The model under review builds one solid part; all positions refer to its coordinate system, in mm. Round coordinates to 2 decimals unless told otherwise and drop trailing zeros. Write each loop counter-clockwise with the first axis right and the second up, starting at its lowest first coordinate (ties: lowest second). Pieces come first, ordered by that corner, then holes. Notation, with made-up numbers: (40, 24) -> (98, 24) arc R14 ccw to (98, 41) -> close; hole circle Ø11 at (35, 86.25). An arc over 180 degrees is marked (long way). Answer as a JSON object with one key per item and string values. Group by question number.
1) We need section A-A, the plane x = -25.75. Write out the cut boundary in (y, z).
2) Mouldability with a two-part tool opening along X and no side actions: class faces 1 (the flat face through (30, 0, 1)), 2 (the flat face through (-14, 14, 2)), 3 (the cylindrical face through (-2.343, -17.847, 0.986)) as pulls with the +X half, pulls with the -X half, needs draft (parallel to the pull), parting line crosses it, or undercut.
3) To check wall thickness, follow probe 1 along Y at (x, z) = (-25.75, 0.5); probe 2 along X at (y, z) = (-26.5, 0.6); probe 3 along Y at (x, z) = (0, 1.4). State the ranges of each line that lie inside material, in increasing order. Write a range as [from, to].
4) We need section B-B, the plane z = 1.25. Write out the cut boundary in (x, y).
5) We need section D-D, the plane x = 0. Write out the cut boundary in (y, z).
Autodesk Fusion 360 part; units mm, degrees
sketch "Sketch1" plane through (0, 0, 0) normal (0, 0, 1) x (1, 0, 0)
  line L0 (-30, 30) -> (30, 30)
  line L1 (30, 30) -> (30, -30)
  line L2 (30, -30) -> (-30, -30)
  line L3 (-30, -30) -> (-30, 30)
  line L4 (-30, 30) -> (30, -30) construction
  line L5 (30, 30) -> (-30, -30) construction
  circle A0 centre (-25.75, 25.75) radius 1.55
  circle A1 centre (25.75, 25.75) radius 1.55
  circle A2 centre (25.76, -25.76) radius 1.55
  circle A3 centre (-25.75, -25.75) radius 1.55
  circle A4 centre (0, 0) radius 18
  dimension "d1" = 60
  dimension "d2" = 60
  dimension "d3" = 3.1
  dimension "d4" = 3.1
  dimension "d5" = 3.1
  dimension "d6" = 3.1
  dimension "d7" = 4.24
  dimension "d8" = 4.25
  dimension "d9" = 4.25
  dimension "d10" = 4.25
  dimension "d11" = 36
extrude "Extrude1" add sketch "Sketch1" along normal blind 2
chamfer "Chamfer1" distance 1.25 angle 45 4 edges at (-27.1951, 26.3105, 2) (24.3049, 26.3105, 2) (24.3149, -25.1995, 2) (-27.1951, -25.1895, 2)
Here are the results:
{
 "1": {"outline": "(-30, 0) -> (-27.3, 0) -> (-27.3, 0.75) -> (-28.55, 2) -> (-30, 2) -> close; (-24.2, 0) -> (24.2, 0) -> (24.2, 0.75) -> (22.95, 2) -> (-22.95, 2) -> (-24.2, 0.75) -> close; (27.3, 0) -> (30, 0) -> (30, 2) -> (28.55, 2) -> (27.3, 0.75) -> close"},
 "2": {"face 1": "pulls with the +X half", "face 2": "needs draft", "face 3": "undercut"},
 "3": {"probe 1": "y = [-30, -27.3], [-24.2, 24.2], [27.3, 30]", "probe 2": "x = [-30, -27.11], [-24.39, 24.4], [27.12, 30]", "probe 3": "y = [-30, -18], [18, 30]"},
 "4": {"outline": "(-30, -30) -> (30, -30) -> (30, 30) -> (-30, 30) -> close; hole circle Ø4.1 at (-25.75, -25.75); hole circle Ø4.1 at (-25.75, 25.75); hole circle Ø36 at (0, 0); hole circle Ø4.1 at (25.75, 25.75); hole circle Ø4.1 at (25.76, -25.76)"},
 "5": {"outline": "(-30, 0) -> (-18, 0) -> (-18, 2) -> (-30, 2) -> close; (18, 0) -> (30, 0) -> (30, 2) -> (18, 2) -> close"}
}
